Autodesk Inventor part; units mm, degrees
ref_plane "YZ Plane" through (0, 0, 0) normal (1, 0, 0) x (0, 1, 0)
ref_plane "XZ Plane" through (0, 0, 0) normal (0, 1, 0) x (-1, 0, 0)
ref_plane "XY Plane" through (0, 0, 0) normal (0, 0, 1) x (1, 0, 0)
sketch "Szkic1" plane through (0, 0, 0) normal (0, 0, 1) x (1, 0, 0)
  line L0 (107.302, 11.5082) -> (232.302, 11.5082)
  line L1 (232.302, 11.5082) -> (232.302, -288.4918)
  line L2 (232.302, -288.4918) -> (107.302, -288.4918)
  line L3 (107.302, -288.4918) -> (107.302, 11.5082)
  point P0 (0, 0)
  dimension "d0" = 125
  dimension "d1" = 300
extrude "Wyciągnięcie proste1" add sketch "Szkic1" along normal blind 20
sketch "Szkic2" plane through (0, 0, 20) normal (0, 0, 1) x (1, 0, 0)
  line L0 (232.302, 11.5082) -> (107.302, 11.5082)
  line L1 (107.302, -288.4918) -> (232.302, -288.4918)
  line L2 (107.302, 11.5082) -> (127.302, 11.5082)
  line L3 (127.302, 11.5082) -> (127.302, -288.4918)
  line L4 (127.302, -288.4918) -> (107.302, -288.4918)
  line L5 (107.302, -288.4918) -> (107.302, 11.5082)
  line L6 (232.302, -288.4918) -> (232.302, 11.5082)
  line L7 (107.302, 11.5082) -> (232.302, 11.5082)
  line L8 (232.302, 11.5082) -> (232.302, -8.4918)
  line L9 (232.302, -8.4918) -> (107.302, -8.4918)
  line L10 (107.302, -8.4918) -> (107.302, 11.5082)
  line L11 (107.302, -288.4918) -> (232.302, -288.4918)
  line L12 (232.302, -288.4918) -> (232.302, -268.4918)
  line L13 (232.302, -268.4918) -> (107.302, -268.4918)
  line L14 (107.302, -268.4918) -> (107.302, -288.4918)
  point P0 (0, 0)
  point P1 (127.302, -8.4918)
  point P2 (127.302, -268.4918)
  dimension "d4" = 20
  dimension "d5" = 20
  dimension "d8" = 20
extrude "Wyciągnięcie proste2" add sketch "Szkic2" along normal blind 60 contours L6 L9 L3 L0 | L3 L9 L5 L0 | L3 L13 L5 L9 | L6 L1 L3 L13 | L3 L1 L5 L13
sketch "Szkic3" plane through (107.302, -288.4918, 0) normal (-1, 0, 0) x (0, 0, 1)
  line L0 (0, 300) -> (80, 300)
  line L1 (0, 0) -> (80, 0)
  line L2 (80, 300) -> (50, 300)
  line L3 (50, 300) -> (50, 0)
  line L4 (50, 0) -> (80, 0)
  line L5 (80, 0) -> (80, 300)
  circle A0 centre (50, 250) radius 10
  circle A1 centre (50, 200) radius 10
  circle A2 centre (50, 50) radius 10
  line L6 (50, 200) -> (50, 50) construction
  line L7 (40, 200) -> (40, 50)
  line L8 (60, 50) -> (60, 200)
  arc A3 (60, 200) -> (40, 200) centre (50, 200) ccw
  arc A4 (40, 50) -> (60, 50) centre (50, 50) ccw
  point P0 (0, 288.4918)
  point P1 (65, 300)
  point P2 (65, 0)
  point P3 (50, 125)
  point P4 (60, 200)
  dimension "d9" = 30
  dimension "d10" = 50
  dimension "d11" = 50
  dimension "d12" = 100
  dimension "d13" = 20
  dimension "d14" = 20
  dimension "d15" = 20
extrude "Wyciągnięcie proste3" cut sketch "Szkic3" against normal through all contours A0 L3 | L3 A0 | A1 L3 | L3 A1 | A2 L3 | L3 A2 | A1 L8 A2 L3 | L3 A2 L7 A1
mirror "Odbij1" about plane through (232.302, -288.4918, 0) normal (1, 0, 0)
properties part number "podstawa"
Design review of the part built by this model. Coordinates are the model's own, in mm. A direction names the side the tool comes from. Round coordinates to 2 decimals unless told otherwise and drop trailing zeros. Loops run counter-clockwise (first coordinate to the right, second up) from the corner with the lowest first, then second, coordinate; pieces in that order, holes last. Notation, with made-up numbers: M 75,15 L 121,15 A28 ccw 121,35 Z; hole C 64.5,75.25 d10. An arc over 180 degrees is marked long. Answer as a JSON object with one key per item and string values.
Item 1: We need section D-D on z = 66.5. Give the boundary of the cut face in (x, y), and give its area (3 significant figures).
Answer sheet:
{"outline": "M 107.3,-288.49 L 357.3,-288.49 L 357.3,11.51 L 107.3,11.51 Z; hole M 127.3,-268.49 L 337.3,-268.49 L 337.3,-8.49 L 127.3,-8.49 Z", "area": "20,400 mm^2"}
Item 2: Machinability: for faces 5 (the flat face through (119, -136, 80)), 6 (the cylindrical face through (347.44, -248.49, 50.22)), 7 (the flat face through (337.302, -140, 36)), which of the approach directions +Z, -Z, +X, -X, +Y, -Y give a long, thin tool a straight path to every point of the face, cutting with its end or side? Answer none if there is none.
Answer sheet:
{"face 5": "+Z, +X, -X, +Y, -Y", "face 6": "+X, -X", "face 7": "+Z"}
Item 3: The part is to be moulded in two halves that separate along Z. For faces 1 (the cylindrical face through (117.16, -38.05, 40.01)), 2 (the flat face through (231, -136, 0)), 3 (the flat face through (117, -162, 40)), 4 (the flat face through (107.302, -141, 39)), say which applies: pulls with the +Z half, pulls with the -Z half, needs draft (parallel to the pull), parting line crosses it, or undercut.
Answer sheet:
{"face 1": "undercut", "face 2": "pulls with the -Z half", "face 3": "undercut", "face 4": "needs draft"}
Item 4: Clearance check with a flat-ended pin moving along its axis: P1, Ø8, axis at x = 184, y = -185.5, coming from the +Z side. State where the tip first meets the part, or that it passes through.
Answer sheet:
{"P1": "stops at z = 20"}
Item 5: We need section B-B on x = 309. Give the boundary of the cut face in (y, z).
Answer sheet:
{"outline": "M -288.49,0 L 11.51,0 L 11.51,80 L -8.49,80 L -8.49,20 L -268.49,20 L -268.49,80 L -288.49,80 Z"}
Item 6: We need section A-A on z = 50. Give the boundary of the cut face in (x, y).
Answer sheet:
{"outline": "M 107.3,-288.49 L 357.3,-288.49 L 357.3,-248.49 L 337.3,-248.49 L 337.3,-268.49 L 127.3,-268.49 L 127.3,-248.49 L 107.3,-248.49 Z; M 107.3,-78.49 L 127.3,-78.49 L 127.3,-48.49 L 107.3,-48.49 Z; M 107.3,-28.49 L 127.3,-28.49 L 127.3,-8.49 L 337.3,-8.49 L 337.3,-28.49 L 357.3,-28.49 L 357.3,11.51 L 107.3,11.51 Z; M 337.3,-78.49 L 357.3,-78.49 L 357.3,-48.49 L 337.3,-48.49 Z"}
Item 7: Wall thickness on L1, parallel to Y at x = 114, z = 50; L2, parallel to Y at x = 324.5, z = 53; L3, parallel to X at y = -98, z = 32.5: over which ranges is each line inside the solid? List them lowest first. Write a range as from..to.
Answer sheet:
{"L1": "y = -288.49..-248.49, -78.49..-48.49, -28.49..11.51", "L2": "y = -288.49..-268.49, -8.49..11.51", "L3": "x = 107.3..127.3, 337.3..357.3"}
Item 8: We need section C-C on y = -60.5. Give the boundary of the cut face in (x, z), and give its area (3 significant figures).
Answer sheet:
{"outline": "M 107.3,0 L 357.3,0 L 357.3,80 L 337.3,80 L 337.3,20 L 127.3,20 L 127.3,80 L 107.3,80 Z", "area": "7,400 mm^2"}
